Can you work these out from the model? Positions are in its coordinate system, mm. A direction names the side the tool comes from. Give positions to 0.01 mm unless a question says otherwise; leave off trailing zeros. Order: outer loops, then holes, each group sorted by start corner. A loop starts at its lowest first (then second) coordinate and runs counter-clockwise, first axis right, second up. Notation, with made-up numbers: M 7.5,-24.5 L 17.5,-24.5 A21 ccw 17.5,-18.5 Z; hole C -18,86.25 d5. An arc over 180 degrees is marked long. Answer as a JSON object with one key per item and string values.
```python
from build123d import *

# Parameters (mm, degrees)
F0_W     = 64
F0_H     = 25.75
F0_R     = 3.625
F1_DEPTH = 6
F3_DEPTH = 26.50399


with BuildPart() as f1:
    # F0 (on Front) → F1 (new body)
    with BuildSketch(Plane.XZ):
        with Locations((-2.422976, 12.875)):
            Rectangle(F0_W, F0_H)
        with Locations((-2.422976, 12.875)):
            Circle(F0_R, mode=Mode.SUBTRACT)
    extrude(amount=F1_DEPTH)

    # F2 (on face) → F3 (cut)
    with BuildSketch(Plane.XY.offset(25.75)):
        Polygon((-34.422976, 0), (-34.422976, -0.7), (-32.922976, 0), align=None)
        Polygon((-32.922976, 0), (-31.422976, -0.7), (-29.922976, 0), align=None)
        Polygon((-29.922976, 0), (-28.422976, -0.7), (-26.922976, 0), align=None)
        Polygon((-26.922976, 0), (-25.422976, -0.7), (-23.922976, 0), align=None)
        Polygon((-23.922976, 0), (-22.422976, -0.7), (-20.922976, 0), align=None)
        Polygon((-20.922976, 0), (-19.422976, -0.7), (-17.922976, 0), align=None)
        Polygon((-17.922976, 0), (-16.422976, -0.7), (-14.922976, 0), align=None)
        Polygon((-14.922976, 0), (-13.422976, -0.7), (-11.922976, 0), align=None)
        Polygon((-11.922976, 0), (-10.422976, -0.7), (-8.922976, 0), align=None)
        Polygon((-8.922976, 0), (-7.422976, -0.7), (-5.922976, 0), align=None)
        Polygon((-5.922976, 0), (-4.422976, -0.7), (-2.922976, 0), align=None)
        Polygon((-2.922976, 0), (-1.422976, -0.7), (0.077024, 0), align=None)
        Polygon((0.077024, 0), (1.577024, -0.7), (3.077024, 0), align=None)
        Polygon((4.577024, -0.7), (6.077024, 0), (3.077024, 0), align=None)
        Polygon((7.577024, -0.7), (9.077024, 0), (6.077024, 0), align=None)
        Polygon((10.577024, -0.7), (12.077024, 0), (9.077024, 0), align=None)
        Polygon((13.577024, -0.7), (15.077024, 0), (12.077024, 0), align=None)
        Polygon((16.577024, -0.7), (18.077024, 0), (15.077024, 0), align=None)
        Polygon((19.577024, -0.7), (21.077024, 0), (18.077024, 0), align=None)
        Polygon((22.577024, -0.7), (24.077024, 0), (21.077024, 0), align=None)
        Polygon((25.577024, -0.7), (27.077024, 0), (24.077024, 0), align=None)
        Polygon((28.577024, -0.7), (29.577024, -0.7), (29.577024, 0), (27.077024, 0), align=None)
    extrude(amount=-F3_DEPTH, mode=Mode.SUBTRACT)


solid = f1.part
```
1) Thinking about a two-plate mould opening in X: for faces 1 (the face through (-5.183, -0.345, 19.868)), 2 (the face through (-33.683, -0.355, 13.055)), 3 (the face through (-0.683, -0.355, 20.697)), which applies, pulls with the +X half, pulls with the -X half, needs draft (parallel to the pull), parting line crosses it, or undercut?
Results found:
{"face 1": "undercut", "face 2": "pulls with the -X half", "face 3": "undercut"}
2) I'm going to push a flat-ended pin straight in: pin 1 Ø0.8 at (x, z) = (29, 15) entering from +Y. Where does the tip first touch, or does it pass through?
Results found:
{"pin 1": "stops at y = -0.7"}
3) For faces 4 (the face through (-6.044, -2.958, 13.034)), 5 (the face through (-30.683, -0.355, 13.055)), which set-ups out of +Z, -Z, +X, -X, +Y, -Y let a thin tool reach every point of the face, with its end or its side?
Results found:
{"face 4": "+Y, -Y", "face 5": "+Z, -Z, +Y"}
4) I want a section at B-B on x = -17. Write out the boundary of the cut face in (y, z), and give its area (3 significant figures).
Results found:
{"outline": "M -6,0 L -0.43,0 L -0.43,25.75 L -6,25.75 Z", "area": "143 mm²"}
5) I want a section at C-C on x = 8.5. Write out the boundary of the cut face in (y, z), and give its area (3 significant figures).
Results found:
{"outline": "M -6,0 L -0.27,0 L -0.27,25.75 L -6,25.75 Z", "area": "148 mm²"}
6) I need wall thicknesses on L1, parallel to X at y = -2, z = 10.5; L2, parallel to Z at x = -1.5, y = -4; L3, parallel to X at y = -4, z = 14.75. Which ranges of each line are inside material? Lowest first, please.
Results found:
{"L1": "x = -34.42 to -5.16, 0.32 to 29.58", "L2": "z = 0 to 9.37, 16.38 to 25.75", "L3": "x = -34.42 to -5.53, 0.68 to 29.58"}
7) I want a section at A-A on y = -1.75. Write out the boundary of the cut face in (x, z) (3 decimals), and give its area (3 significant figures).
Results found:
{"outline": "M -34.423,0 L 29.577,0 L 29.577,25.75 L -34.423,25.75 Z; hole C -2.423,12.875 d7.25", "area": "1,610 mm²"}
